Verification items for the finished model (mm, model axes). Round coordinates to 2 decimals unless told otherwise and drop trailing zeros. Write each loop counter-clockwise with the first axis right and the second up, starting at its lowest first coordinate (ties: lowest second). Pieces come first, ordered by that corner, then holes.
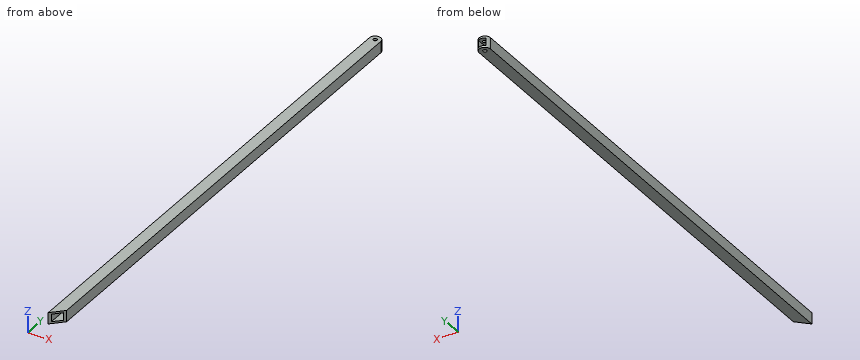
from build123d import *

# Parameters (mm, degrees)
ESQUISSE1_R             = 3.175
BOSS_EXTRU_1_DEPTH      = 19.05
ESQUISSE2_W             = 12.7
ESQUISSE2_H             = 12.7
ENL_V_MAT_EXTRU_3_DEPTH = 871


with BuildPart() as part:
    # Esquisse1 → Boss.-Extru.1 (new body)
    with BuildSketch(Plane.XY):
        with BuildLine():
            Line((0, 0), (19.05, 19.05))
            Line((19.05, 19.05), (19.05, 860.475))
            ThreePointArc((19.05, 860.475), (9.525, 870), (0, 860.475))
            Line((0, 860.475), (0, 0))
        make_face()
        with Locations((9.525, 860.475)):
            Circle(ESQUISSE1_R, mode=Mode.SUBTRACT)
    extrude(amount=BOSS_EXTRU_1_DEPTH)

    # Esquisse2 → Enlèv. mat.-Extru.3 (cut, through all)
    with BuildSketch(Plane(origin=(0, 0, 0), x_dir=(1, 0, 0), z_dir=(0, 1, 0))):
        with Locations((9.525, -9.525)):
            Rectangle(ESQUISSE2_W, ESQUISSE2_H)
    extrude(amount=ENL_V_MAT_EXTRU_3_DEPTH, mode=Mode.SUBTRACT)


solid = part.part
Q1. Material ranges on line 1 along Z through (x, y) = (7.5, 270.5) (3 decimals); line 2 along Y through (x, z) = (12, 18), recorded low to high.
Recorded:
line 1: z = 0 to 3.175, 15.875 to 19.05
line 2: y = 12 to 858.49, 862.46 to 869.67
Q2. Sectioned sample at B-B (x = 9.5). Enter the section's corners in (y, z) (3 decimals).
Recorded:
outline: (9.5, 0) - (857.3, 0) - (857.3, 3.175) - (9.5, 3.175) - close; (9.5, 15.875) - (857.3, 15.875) - (857.3, 19.05) - (9.5, 19.05) - close; (863.65, 0) - (870, 0) - (870, 3.175) - (863.65, 3.175) - close; (863.65, 15.875) - (870, 15.875) - (870, 19.05) - (863.65, 19.05) - close
Q3. Depth check by flat-ended pin: P1, Ø3, axis at x = 7, z = 15.5, coming from the +Y side; P2, Ø4, axis at x = 9.5, z = 2, coming from the -Y side; P3, Ø2, axis at x = 16, z = 5.5, coming from the -Y side (3 decimals). Enter the tip coordinate at first touch or a pass-through.
Recorded:
P1: stops at y = 869.94
P2: stops at y = 7.5
P3: stops at y = 15.875
Q4. Sectioned sample at C-C (y = 56). Enter the section's corners in (x, z) (3 decimals), plus the area to 3 significant figures.
Recorded:
outline: (0, 0) - (19.05, 0) - (19.05, 19.05) - (0, 19.05) - close; hole (3.175, 3.175) - (15.875, 3.175) - (15.875, 15.875) - (3.175, 15.875) - close
area: 202 mm2
Q5. Sectioned sample at A-A (z = 12). Enter the section's corners in (x, y) (3 decimals).
Recorded:
outline: (0, 0) - (3.175, 3.175) - (3.175, 867.575) arc R9.525 ccw to (0, 860.475) - close; (15.875, 15.875) - (19.05, 19.05) - (19.05, 860.475) arc R9.525 ccw to (15.875, 867.575) - close
